Geometry check sheet. Reference: the model listing, model coordinates, mm. Face numbers are marked on the shaded views. A direction names the side the tool comes from. Coordinates: 2 decimals unless noted, no trailing zeros. Order: outer loops, then holes, each group sorted by start corner. A loop starts at its lowest first (then second) coordinate and runs counter-clockwise, first axis right, second up. Notation, with made-up numbers: M 80.25,87 L 93.25,87 A10 ccw 93.25,105 Z; hole C -6,43 d11. An arc over 180 degrees is marked long. One line per item, written item: value. Start each with the question number.
1) Sectioned sample at A-A, the plane x = 42. Enter the section's corners in (y, z), then the cut area to 3 significant figures.
2) Access from +Z, -Z, +X, -X, +Y, -Y to the whole of each face (thin tool, end or side, straight path). Record for the marked faces 1 and 2.
3) Go/stop test with flat-tipped pins: P1, Ø1.5, axis at x = 37, y = 0.5, coming from the +Z side; P2, Ø2, axis at x = 18.5, z = -0.5, coming from the -Y side. Record where each tip stops, or that it passes through.
4) Thickness scan on L1, parallel to X at y = 4.75, z = -1.5; L2, parallel to Y at x = 28, z = 1; L3, parallel to Y at x = 47.5, z = 0.25. Record the ranges inside material, lowest first. Write a range as from..to.
```python
from build123d import *

# Parameters (mm, degrees)
BASEHEAD_DEPTH  = 4
THDSCHPAT_COUNT = 15
THDSCHPAT_PITCH = 0.666666667


with BuildPart() as part:
    # Sketch1 → BaseHead (new body)
    with BuildSketch(Plane(origin=(0, 0, 0), x_dir=(0, 0, -1), z_dir=(1, 0, 0))):
        Polygon((5, 2.886751346), (5, -2.886751346), (0, -5.773502692), (-5, -2.886751346), (-5, 2.886751346), (0, 5.773502692), align=None)
    extrude(amount=BASEHEAD_DEPTH)

    # BodySke → BaseBody (revolve)
    with BuildSketch(Plane.XY):
        Polygon((0, 0), (60, 0), (60, 2.4455), (59.4455, 3), (0, 3), align=None)
    revolve(axis=Axis((0, 0, 0), (1, 0, 0)))

    # Sketch3 → HeadChamfer (revolve, cut)
    with BuildSketch(Plane.XY):
        Polygon((0, 5), (3.333333333, 10.773502692), (3.333333333, 15.773502692), (-10, 15.773502692), (-10, 5), align=None)
    revolve(axis=Axis((0, 0, 0), (1, 0, 0)), mode=Mode.SUBTRACT)

    # ThdSchSke → ThreadSchematic (revolve, cut)
    with BuildSketch(Plane.XY):
        Polygon((50, -2.4455), (49.61173492, -3), (49.61173492, -3.75), (50.38826508, -3.75), (50.38826508, -3), align=None)
    threadschematic = revolve(axis=Axis((-3.175, 0, 0), (1, 0, 0)), mode=Mode.SUBTRACT)

    # ThdSchPat: ThreadSchematic ×15
    with Locations(*[(i * THDSCHPAT_PITCH, 0, 0) for i in range(1, THDSCHPAT_COUNT)]):
        add(threadschematic, mode=Mode.SUBTRACT)


solid = part.part
```
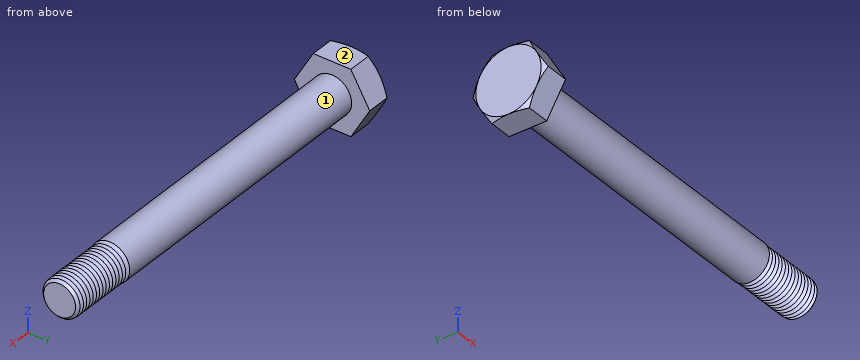
Final values:
1. outline: C 0,0 d6
1. area: 28.3 mm^2
2. face 1: +X
2. face 2: +Z, +X, -X, +Y, -Y
3. P1: stops at z = 3
3. P2: stops at y = -3
4. L1: x = 0..4
4. L2: y = -2.83..2.83
4. L3: y = -2.99..2.99
